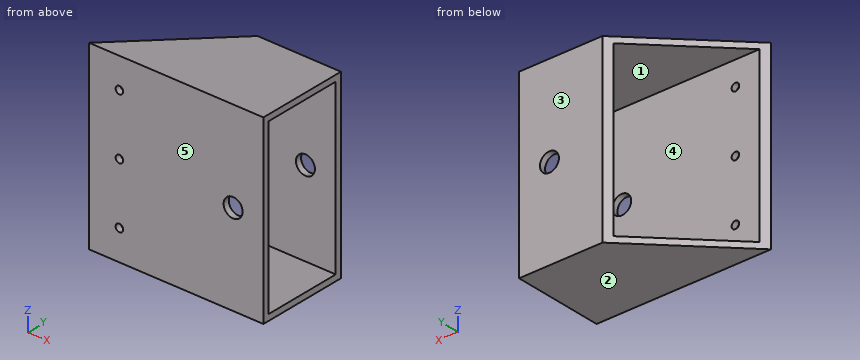
```python
from build123d import *

# Parameters (mm, degrees)
SKETCH1_W           = 76.2
SKETCH1_H           = 38.1
SKETCH1_W_2         = 71.12
SKETCH1_H_2         = 33.02
EXTRUDE_THIN1_DEPTH = 101.6
SKETCH7_R           = 3.9751
CUT_EXTRUDE6_DEPTH  = 39.1
SKETCH10_W          = 76.2
SKETCH10_H          = 38.1
CUT_EXTRUDE9_DEPTH  = 28.575
CUT_EXTRUDE10_DEPTH = 77.2
SKETCH9_R           = 1.5875
CUT_EXTRUDE11_DEPTH = 3.54


with BuildPart() as part:
    # Sketch1 → Extrude-Thin1 (new body)
    with BuildSketch(Plane(origin=(0, 0, 0), x_dir=(0, 0, -1), z_dir=(1, 0, 0))):
        Rectangle(SKETCH1_W, SKETCH1_H)
        Rectangle(SKETCH1_W_2, SKETCH1_H_2, mode=Mode.SUBTRACT)
    extrude(amount=EXTRUDE_THIN1_DEPTH)

    # Sketch7 → Cut-Extrude6 (cut, through all)
    with BuildSketch(Plane(origin=(0, 19.05, 0), x_dir=(1, 0, 0), z_dir=(0, 1, 0))):
        with Locations((88.9, 0)):
            Circle(SKETCH7_R)
    extrude(amount=-CUT_EXTRUDE6_DEPTH, mode=Mode.SUBTRACT)

    # Sketch10 → Cut-Extrude9 (cut)
    with BuildSketch(Plane.ZY):
        Rectangle(SKETCH10_W, SKETCH10_H)
    extrude(amount=-CUT_EXTRUDE9_DEPTH, mode=Mode.SUBTRACT)

    # Sketch11 → Cut-Extrude10 (cut, through all)
    with BuildSketch(Plane(origin=(0, 0, -38.1), x_dir=(-1, 0, 0), z_dir=(0, 0, -1))):
        Polygon((-28.575, -19.05), (-66.675, 19.05), (-28.575, 19.05), align=None)
    extrude(amount=-CUT_EXTRUDE10_DEPTH, mode=Mode.SUBTRACT)

    # Sketch9 → Cut-Extrude11 (cut, through all)
    with BuildSketch(Plane(origin=(0, -16.51, 0), x_dir=(1, 0, 0), z_dir=(0, 1, 0))):
        with Locations((41.275, 0)):
            Circle(SKETCH9_R)
        with Locations((41.275, -25.4)):
            Circle(SKETCH9_R)
        with Locations((41.275, 25.4)):
            Circle(SKETCH9_R)
    extrude(amount=-CUT_EXTRUDE11_DEPTH, mode=Mode.SUBTRACT)


solid = part.part
```
The listing builds one solid part. Answer for the finished solid, in the listing's coordinates (mm). Face numbers are marked on the shaded views. A direction names the side the tool comes from. Round coordinates to 2 decimals unless told otherwise and drop trailing zeros. Order: outer loops, then holes, each group sorted by start corner. A loop starts at its lowest first (then second) coordinate and runs counter-clockwise, first axis right, second up. Notation, with made-up numbers: (-18.5, 69.25) - (10.5, 69.25) arc R23 ccw to (10.5, 100.25) - close; hole circle Ø9 at (71, 20.25). An arc over 180 degrees is marked (long way). Put each result on its own line as item: value. Start each with the question number.
(1) Given P1, Ø3.5, axis at x = 41.275, z = -25.4, coming from the +Y side; P2, Ø1.9, axis at x = 41.275, z = 25.4, coming from the -Y side, each flat-ended and moving along its own axis, determine where each tip first touches the part or whether it passes through.
(2) For the marked faces 4 and 5, determine the directions among +Z, -Z, +X, -X, +Y, -Y from which every point of the face is accessible in a straight line to the end or side of a thin tool.
(3) Find section C-C (y = 13.5). Give the vertices of the cut face in (x, z) (3 decimals), plus the area to 3 significant figures.
(4) Straight lines are drawn through the part: probe 1 along Y at (x, z) = (88.5, 10); probe 2 along Z at (x, y) = (43.5, -6.5); probe 3 along Z at (x, y) = (88.9, -18.15). For each, find the intervals that lie inside material, in ascending order. Write a range as from..to.
(5) Find section A-A (z = 5.5). Give the vertices of the cut face in (x, y) (3 decimals).
(6) Find section B-B (x = 88.9). Give the vertices of the cut face in (y, z), plus the area to 3 significant figures.
(7) Find section D-D (x = 41.5). Give the vertices of the cut face in (y, z) (3 decimals).
(8) Determine the mould class of the marked faces 1, 2 and 3 for opening direction Y: released by +Y, released by -Y, zero draft, split by the parting line, or undercut.
Reply:
1. P1: y = -16.51
1. P2: through
2. face 4: +X, -X
2. face 5: +Z, -Z, +X, -X, -Y
3. outline: (61.125, -38.1) - (101.6, -38.1) - (101.6, -35.56) - (61.125, -35.56) - close; (61.125, 35.56) - (101.6, 35.56) - (101.6, 38.1) - (61.125, 38.1) - close
3. area: 206 mm^2
4. probe 1: -19.05..-16.51, 16.51..19.05
4. probe 2: -38.1..-35.56, 35.56..38.1
4. probe 3: -38.1..-3.98, 3.98..38.1
5. outline: (28.575, -19.05) - (101.6, -19.05) - (101.6, -16.51) - (31.115, -16.51) - close; (64.135, 16.51) - (101.6, 16.51) - (101.6, 19.05) - (66.675, 19.05) - close
6. outline: (-19.05, -38.1) - (19.05, -38.1) - (19.05, -3.98) - (16.51, -3.98) - (16.51, -35.56) - (-16.51, -35.56) - (-16.51, -3.98) - (-19.05, -3.98) - close; (-19.05, 3.98) - (-16.51, 3.98) - (-16.51, 35.56) - (16.51, 35.56) - (16.51, 3.98) - (19.05, 3.98) - (19.05, 38.1) - (-19.05, 38.1) - close
6. area: 514 mm^2
7. outline: (-19.05, -38.1) - (-6.125, -38.1) - (-6.125, -35.56) - (-16.51, -35.56) - (-16.51, -26.971) - (-19.05, -26.971) - close; (-19.05, -23.829) - (-16.51, -23.829) - (-16.51, -1.571) - (-19.05, -1.571) - close; (-19.05, 1.571) - (-16.51, 1.571) - (-16.51, 23.829) - (-19.05, 23.829) - close; (-19.05, 26.971) - (-16.51, 26.971) - (-16.51, 35.56) - (-6.125, 35.56) - (-6.125, 38.1) - (-19.05, 38.1) - close
8. face 1: undercut
8. face 2: zero draft
8. face 3: released by +Y
